Could you check a few things on this drawing? It's one solid part, dimensions in mm from its lowest x, y, z. A direction names the side the tool comes from. Round coordinates to 2 decimals unless told otherwise and drop trailing zeros. Loops run counter-clockwise (first coordinate to the right, second up) from the corner with the lowest first, then second, coordinate; pieces in that order, holes last. Notation, with made-up numbers: (-26, 77) -> (-4, 77) arc R10 cw to (-4, 83) -> close; hole circle Ø8 at (31, 73.25). An arc over 180 degrees is marked (long way). Write each question's results on one line, items separated by ' | '.
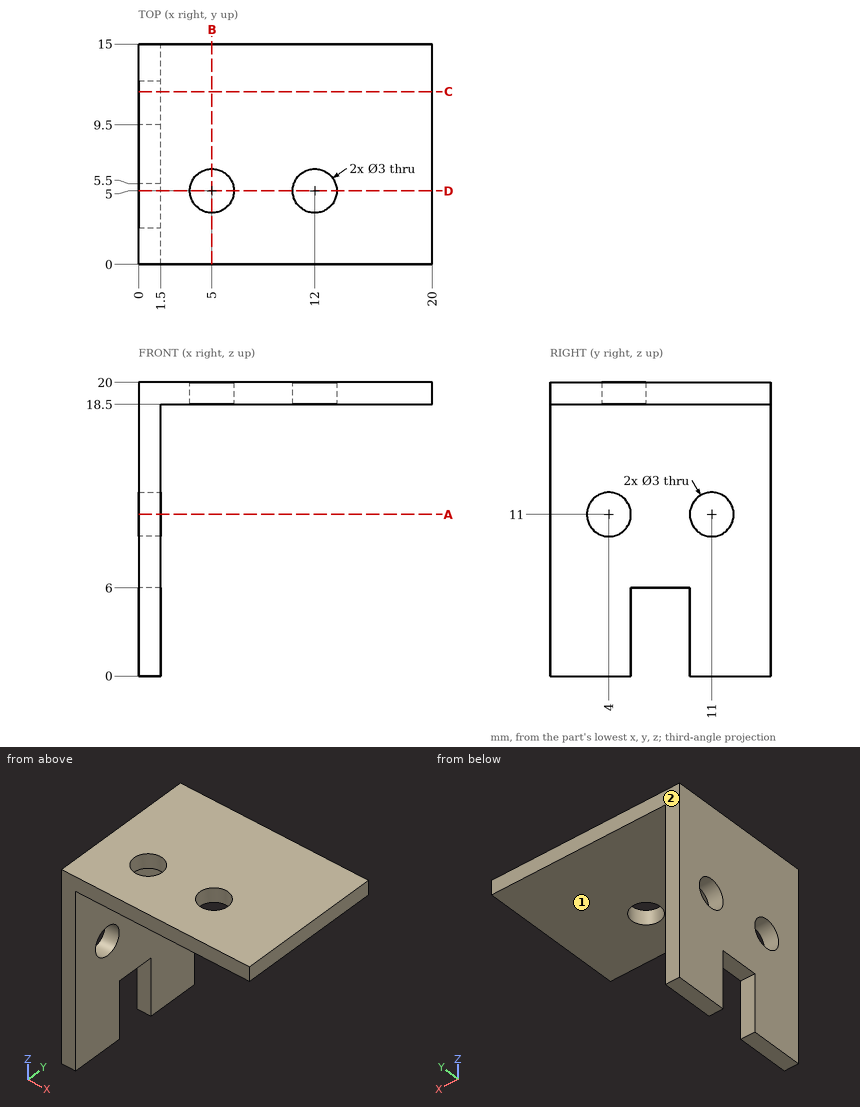
1) I need wall thicknesses on line 1 (Y direction, x = 0.4, z = 11); line 2 (Y direction, x = 5, z = 19.05); line 3 (X direction, y = 5.5, z = 15.25). Which ranges of each line are inside material? Lowest first, please.
Model answer:
line 1: y = 0 to 2.5, 5.5 to 9.5, 12.5 to 15 | line 2: y = 0 to 3.5, 6.5 to 15 | line 3: x = 0 to 1.5
2) I want a section at B-B, the plane x = 5. Write out the boundary of the cut face in (y, z).
Model answer:
outline: (0, 18.5) -> (3.5, 18.5) -> (3.5, 20) -> (0, 20) -> close; (6.5, 18.5) -> (15, 18.5) -> (15, 20) -> (6.5, 20) -> close
3) I want a section at D-D, the plane y = 5. Write out the boundary of the cut face in (x, z).
Model answer:
outline: (0, 0) -> (1.5, 0) -> (1.5, 9.88) -> (0, 9.88) -> close; (0, 12.12) -> (1.5, 12.12) -> (1.5, 18.5) -> (3.5, 18.5) -> (3.5, 20) -> (0, 20) -> close; (6.5, 18.5) -> (10.5, 18.5) -> (10.5, 20) -> (6.5, 20) -> close; (13.5, 18.5) -> (20, 18.5) -> (20, 20) -> (13.5, 20) -> close
4) For the marked faces 1 and 2, which set-ups out of +Z, -Z, +X, -X, +Y, -Y let a thin tool reach every point of the face, with its end or its side?
Model answer:
face 1: -Z, +X, +Y, -Y | face 2: +Z, -Z, +X, -X, +Y
5) I'm going to push flat-ended pins straight in: pin 1 (5 mm diameter, centred on x = 14, y = 6, fed in from -Z); pin 2 (10 mm diameter, centred on x = 8, z = 11, fed in from +Y); pin 3 (3.5 mm diameter, centred on y = 11, z = 11, fed in from +X). Where does each tip first touch, or does it pass through?
Model answer:
pin 1: stops at z = 18.5 | pin 2: passes through | pin 3: stops at x = 1.5
6) I want a section at C-C, the plane y = 11.75. Write out the boundary of the cut face in (x, z).
Model answer:
outline: (0, 0) -> (1.5, 0) -> (1.5, 9.7) -> (0, 9.7) -> close; (0, 12.3) -> (1.5, 12.3) -> (1.5, 18.5) -> (20, 18.5) -> (20, 20) -> (0, 20) -> close
7) I want a section at A-A, the plane z = 11. Write out the boundary of the cut face in (x, y), plus the area to 3 significant figures.
Model answer:
outline: (0, 0) -> (1.5, 0) -> (1.5, 2.5) -> (0, 2.5) -> close; (0, 5.5) -> (1.5, 5.5) -> (1.5, 9.5) -> (0, 9.5) -> close; (0, 12.5) -> (1.5, 12.5) -> (1.5, 15) -> (0, 15) -> close | area: 13.5 mm2
